from build123d import *

# Parameters (mm, degrees)
SZKIC1_W                    = 20
SZKIC1_H                    = 20
DODANIE_WYCI_GNI_CIE1_DEPTH = 20
SZKIC2_W                    = 15.7
SZKIC2_H                    = 15.7
DODANIE_WYCI_GNI_CIE2_DEPTH = 4.28
SZKIC3_W                    = 15.662415204
SZKIC3_H                    = 15.662415203
DODANIE_WYCI_GNI_CIE3_DEPTH = 4.28
SZKIC4_W                    = 15.662415203
SZKIC4_H                    = 15.662415203
DODANIE_WYCI_GNI_CIE4_DEPTH = 4.28
SZKIC5_W                    = 17.455323011
SZKIC5_H                    = 17.455323012
DODANIE_WYCI_GNI_CIE5_DEPTH = 25.72
SZKIC6_W                    = 17.458466428
SZKIC6_H                    = 17.458466428
DODANIE_WYCI_GNI_CIE6_DEPTH = 25.72
SZKIC7_W                    = 17.458466427
SZKIC7_H                    = 17.458466428
DODANIE_WYCI_GNI_CIE7_DEPTH = 25.72
ZAOKR_GLENIE2_R             = 1


with BuildPart() as part:
    # Szkic1 → Dodanie-wyciągnięcie1 (new body)
    with BuildSketch(Plane.XY):
        with Locations((-3.917212592, 19.226146443)):
            Rectangle(SZKIC1_W, SZKIC1_H)
    extrude(amount=DODANIE_WYCI_GNI_CIE1_DEPTH)

    # Szkic2 → Dodanie-wyciągnięcie2 (add)
    with BuildSketch(Plane(origin=(0, 29.226146443, 0), x_dir=(1, 0, 0), z_dir=(0, 1, 0))):
        with Locations((-3.957055084, -10.078566334)):
            Rectangle(SZKIC2_W, SZKIC2_H)
    extrude(amount=DODANIE_WYCI_GNI_CIE2_DEPTH)

    # Szkic3 → Dodanie-wyciągnięcie3 (add)
    with BuildSketch(Plane(origin=(6.082787408, 0, 0), x_dir=(0, 0, -1), z_dir=(1, 0, 0))):
        with Locations((-10, 19.226146442)):
            Rectangle(SZKIC3_W, SZKIC3_H)
    extrude(amount=DODANIE_WYCI_GNI_CIE3_DEPTH)

    # Szkic4 → Dodanie-wyciągnięcie4 (add)
    with BuildSketch(Plane(origin=(0, 0, 0), x_dir=(-1, 0, 0), z_dir=(0, 0, -1))):
        with Locations((3.917212592, 19.226146442)):
            Rectangle(SZKIC4_W, SZKIC4_H)
    extrude(amount=DODANIE_WYCI_GNI_CIE4_DEPTH)

    # Szkic5 → Dodanie-wyciągnięcie5 (add)
    with BuildSketch(Plane(origin=(0, 0, -4.28), x_dir=(-1, 0, 0), z_dir=(0, 0, -1))):
        with Locations((4.144874098, 18.998484937)):
            Rectangle(SZKIC5_W, SZKIC5_H)
    extrude(amount=DODANIE_WYCI_GNI_CIE5_DEPTH)

    # Szkic6 → Dodanie-wyciągnięcie6 (add)
    with BuildSketch(Plane(origin=(10.362787408, 0, 0), x_dir=(0, 0, -1), z_dir=(1, 0, 0))):
        with Locations((-10, 19.226146443)):
            Rectangle(SZKIC6_W, SZKIC6_H)
    extrude(amount=DODANIE_WYCI_GNI_CIE6_DEPTH)

    # Szkic7 → Dodanie-wyciągnięcie7 (add)
    with BuildSketch(Plane(origin=(0, 33.506146443, 0), x_dir=(1, 0, 0), z_dir=(0, 1, 0))):
        with Locations((-3.957055085, -10.078566334)):
            Rectangle(SZKIC7_W, SZKIC7_H)
    extrude(amount=DODANIE_WYCI_GNI_CIE7_DEPTH)

    # Zaokrąglenie2
    zaokr_glenie2_edges = [part.edges().sort_by_distance(p)[0] for p in [
        (4.582787408, 27.726146443, -17.14),
        (4.582787408, 10.270823431, -17.14),
        (-12.872535603, 10.270823431, -17.14),
        (-12.872535603, 27.726146443, -17.14),
        (23.222787408, 10.496913229, 18.729233214),
        (23.222787408, 10.496913229, 1.270766786),
        (23.222787408, 27.955379657, 1.270766786),
        (23.222787408, 27.955379657, 18.729233214),
        (4.772178129, 46.366146443, 18.807799548),
        (4.772178129, 46.366146443, 1.34933312),
        (-12.686288298, 46.366146443, 1.34933312),
        (-12.686288298, 46.366146443, 18.807799548),
    ]]
    fillet(zaokr_glenie2_edges, radius=ZAOKR_GLENIE2_R)


solid = part.part
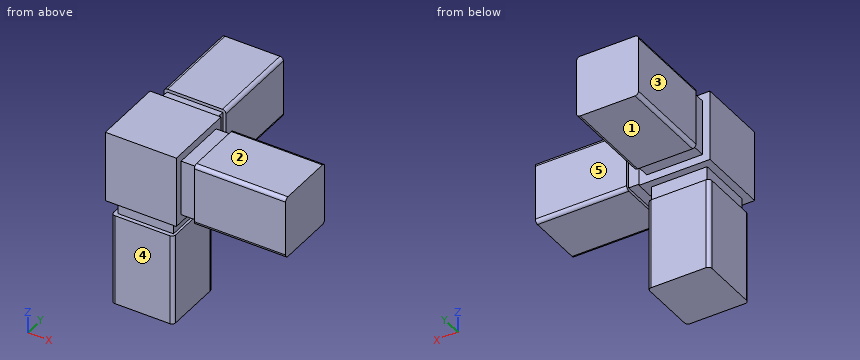
Read the model definition and answer for the solid it produces. Units are mm, in the model's axes. Face numbers are marked on the shaded views. A direction names the side the tool comes from. Round coordinates to 2 decimals unless told otherwise and drop trailing zeros. Order: outer loops, then holes, each group sorted by start corner. A loop starts at its lowest first (then second) coordinate and runs counter-clockwise, first axis right, second up. Notation, with made-up numbers: (-12, 31) - (-4, 31) arc R17 cw to (-4, 42) - close; hole circle Ø8 at (61, 36.5). An arc over 180 degrees is marked (long way). Use one line per item in the form item = value. Start each with the question number.
(1) The part is cut by section B-B (z = -15). Give the vertices of the cut face in (x, y).
(2) Flat-ended cylindrical pins translate along their axes: pin 1 Ø4.5 at (y, z) = (31, 8.5) entering from -X; pin 2 Ø4.5 at (x, y) = (8.5, 20.5) entering from +Z; pin 3 Ø3.5 at (x, y) = (7.5, 18.5) entering from -Z; pin 4 Ø2 at (x, z) = (8, 6) entering from +Y. Find the tip coordinate at first contact, or state that the pin passes through.
(3) Find the intervals of material crossed by line 1 along X through (y, z) = (20, 1.5); line 2 along Y through (x, z) = (23, 5.5); line 3 along X through (y, z) = (19.5, -17), in increasing order. Write a range as from..to.
(4) The part is cut by section C-C (y = 20). Give the vertices of the cut face in (x, z).
(5) The part is cut by section A-A (x = 14). Give the vertices of the cut face in (y, z).
(6) For the marked faces 1, 2, 3, 4 and 5, determine the directions among +Z, -Z, +X, -X, +Y, -Y from which every point of the face is accessible in a straight line to the end or side of a thin tool.
(7) The part is cut by section D-D (x = -1). Give the vertices of the cut face in (y, z), then the cut area to 3 significant figures.
Checked values:
q1.outline = (-12.87, 11.27) arc R1 ccw to (-11.87, 10.27) - (3.58, 10.27) arc R1 ccw to (4.58, 11.27) - (4.58, 26.73) arc R1 ccw to (3.58, 27.73) - (-11.87, 27.73) arc R1 ccw to (-12.87, 26.73) - close
q2.pin_1 = -13.92
q2.pin_2 = 18.73
q2.pin_3 = 0
q2.pin_4 = 27.06
q3.line_1 = -13.92..6.08, 10.36..36.08
q3.line_2 = 10.5..27.96
q3.line_3 = -12.87..4.58
q4.outline = (-13.92, 0) - (-11.75, 0) - (-11.75, -4.28) - (-12.87, -4.28) - (-12.87, -30) - (4.58, -30) - (4.58, -4.28) - (3.91, -4.28) - (3.91, 0) - (6.08, 0) - (6.08, 2.17) - (10.36, 2.17) - (10.36, 1.27) - (36.08, 1.27) - (36.08, 18.73) - (10.36, 18.73) - (10.36, 17.83) - (6.08, 17.83) - (6.08, 20) - (-13.92, 20) - close
q5.outline = (10.5, 2.27) arc R1 ccw to (11.5, 1.27) - (26.96, 1.27) arc R1 ccw to (27.96, 2.27) - (27.96, 17.73) arc R1 ccw to (26.96, 18.73) - (11.5, 18.73) arc R1 ccw to (10.5, 17.73) - close
q6.face_1 = -Z, +X, -X, +Y
q6.face_2 = +Z, +X, +Y, -Y
q6.face_3 = +Z, -Z, -X, +Y
q6.face_4 = -Z, +X, -X, -Y
q6.face_5 = +Z, -Z, +X, +Y
q7.outline = (9.23, 0) - (11.39, 0) - (11.39, -4.28) - (10.27, -4.28) - (10.27, -30) - (27.73, -30) - (27.73, -4.28) - (27.06, -4.28) - (27.06, 0) - (29.23, 0) - (29.23, 2.23) - (33.51, 2.23) - (33.51, 1.35) - (59.23, 1.35) - (59.23, 18.81) - (33.51, 18.81) - (33.51, 17.93) - (29.23, 17.93) - (29.23, 20) - (9.23, 20) - close
q7.area = 1,430 mm^2
